Here's how the part is built. I have some questions about the finished solid (model axes, mm). Face numbers are marked on the shaded views. Give positions to 0.01 mm unless a question says otherwise; leave off trailing zeros. Loops run counter-clockwise (first coordinate to the right, second up) from the corner with the lowest first, then second, coordinate; pieces in that order, holes last. Notation, with made-up numbers: (16.5, -9) -> (51.5, -9) arc R25 ccw to (51.5, 27) -> close; hole circle Ø9 at (-23, -19.75). An arc over 180 degrees is marked (long way). Answer in a Markdown table with one row per item. Add a question column.
Item 1: If we section it at D-D (z = 44): Write out the boundary of the cut face in (x, y).
Item 2: If we section it at C-C (z = -41): Write out the boundary of the cut face in (x, y).
Item 3: If I drill on line 1 (X direction, y = 1.8, z = 0); line 2 (Z direction, x = 350, y = 3.2); line 3 (X direction, y = 2.85, z = 22.5), over which ranges is the centre line in solid material (lowest first)?
Item 4: For P1, Ø4, axis at x = 49, z = -18, coming from the -Y side; P2, Ø9, axis at x = 0, z = 0, coming from the -Y side; P3, Ø1, axis at y = 2.5, z = 11, coming from the -X side, each with a flat end and sliding along its axis, tell me the tip position at first contact or that it passes through.
Item 5: We'd pull the mould along Y, two halves only. Please class the marked faces 1 and 2: released by +Y, released by -Y, zero draft, split by the parting line, or undercut.
Item 6: If we section it at A-A (z = 0): Write out the boundary of the cut face in (x, y).
Item 7: If we section it at B-B (y = 4.15): Give the number of separate pieces and of enclosed holes in the cut face, then the cut area to 3 significant figures.
```python
from build123d import *

# Parameters (mm, degrees)
SKETCH1_R           = 5
SKETCH1_R_2         = 3.5
BOSS_EXTRUDE1_DEPTH = 5
SKETCH2_R           = 3.5
SKETCH2_R_2         = 2.25
SKETCH2_R_3         = 5
CUT_EXTRUDE1_DEPTH  = 5


with BuildPart() as part:
    # Sketch1 → Boss-Extrude1 (new body)
    with BuildSketch(Plane(origin=(0, 0, 0), x_dir=(1, 0, 0), z_dir=(0, 1, 0))):
        with BuildLine():
            Line((0, 50), (350, 50))
            ThreePointArc((350, 50), (400, 0), (350, -50))
            Line((350, -50), (0, -50))
            ThreePointArc((0, -50), (-50, 0), (0, 50))
        make_face()
        with Locations(Location((0, 0, 0), (0, 0, 270))):
            Circle(SKETCH1_R, mode=Mode.SUBTRACT)
        with Locations(Location((350, 0, 0), (0, 0, 270))):
            Circle(SKETCH1_R, mode=Mode.SUBTRACT)
        with Locations(Location((0, 22.5, 0), (0, 0, 270))):
            Circle(SKETCH1_R_2, mode=Mode.SUBTRACT)
        with Locations(Location((350, 22.5, 0), (0, 0, 270))):
            Circle(SKETCH1_R_2, mode=Mode.SUBTRACT)
        with Locations(Location((350, -22.5, 0), (0, 0, 90))):
            Circle(SKETCH1_R_2, mode=Mode.SUBTRACT)
        with Locations(Location((0, -22.5, 0), (0, 0, 90))):
            Circle(SKETCH1_R_2, mode=Mode.SUBTRACT)
    extrude(amount=BOSS_EXTRUDE1_DEPTH)

    # Sketch2 → Cut-Extrude1 (cut)
    with BuildSketch(Plane(origin=(0, 5, 0), x_dir=(1, 0, 0), z_dir=(0, 1, 0))):
        with Locations(Location((205, 22.5, 0), (0, 0, 270))):
            Circle(SKETCH2_R)
        with Locations(Location((15, -30, 0), (0, 0, 270))):
            Circle(SKETCH2_R_2)
        with Locations(Location((105, -30, 0), (0, 0, 270))):
            Circle(SKETCH2_R_2)
        with Locations(Location((105, 30, 0), (0, 0, 270))):
            Circle(SKETCH2_R_2)
        with Locations(Location((15, 30, 0), (0, 0, 270))):
            Circle(SKETCH2_R_2)
        with Locations(Location((205, 0, 0), (0, 0, 270))):
            Circle(SKETCH2_R_3)
        with Locations(Location((205, -22.5, 0), (0, 0, 270))):
            Circle(SKETCH2_R)
    extrude(amount=-CUT_EXTRUDE1_DEPTH, mode=Mode.SUBTRACT)


solid = part.part
```
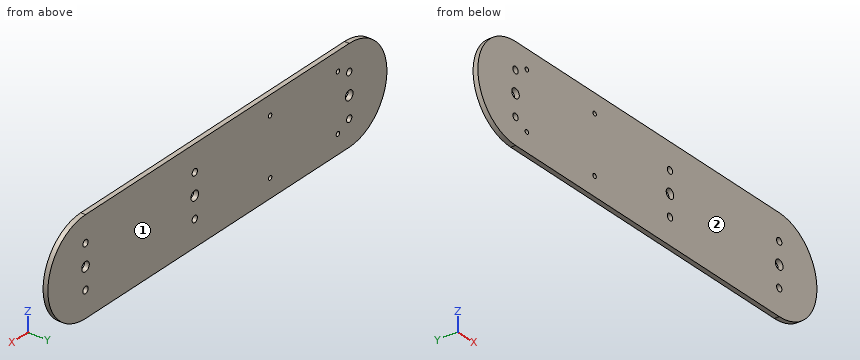
Recorded:
| question | item | result |
|---|---|---|
| 1 | outline | (-23.75, 0) -> (373.75, 0) -> (373.75, 5) -> (-23.75, 5) -> close |
| 2 | outline | (-28.62, 0) -> (378.62, 0) -> (378.62, 5) -> (-28.62, 5) -> close |
| 3 | line 1 | x = -50 to -5, 5 to 200, 210 to 345, 355 to 400 |
| 3 | line 2 | z = -50 to -26, -19 to -5, 5 to 19, 26 to 50 |
| 3 | line 3 | x = -44.65 to -3.5, 3.5 to 201.5, 208.5 to 346.5, 353.5 to 394.65 |
| 4 | P1 | stops at y = 0 |
| 4 | P2 | passes through |
| 4 | P3 | stops at x = -48.89 |
| 5 | face 1 | released by +Y |
| 5 | face 2 | released by -Y |
| 6 | outline | (-50, 0) -> (-5, 0) -> (-5, 5) -> (-50, 5) -> close; (5, 0) -> (200, 0) -> (200, 5) -> (5, 5) -> close; (210, 0) -> (345, 0) -> (345, 5) -> (210, 5) -> close; (355, 0) -> (400, 0) -> (400, 5) -> (355, 5) -> close |
| 7 | separate pieces | 1 |
| 7 | enclosed holes | 13 |
| 7 | area | 42,300 mm^2 |
